The listing builds one solid part. Answer for the finished solid, in the listing's coordinates (mm). Face numbers are marked on the shaded views. A direction names the side the tool comes from. Round coordinates to 2 decimals unless told otherwise and drop trailing zeros. Loops run counter-clockwise (first coordinate to the right, second up) from the corner with the lowest first, then second, coordinate; pieces in that order, holes last. Notation, with made-up numbers: (48.5, -6.5) - (58.5, -6.5) arc R22 ccw to (58.5, 28.5) - close; hole circle Ø3 at (-33, 55). An arc over 180 degrees is marked (long way). One line per question, with ' | ' between items. Start each with the question number.
from build123d import *

# Parameters (mm, degrees)
ESBO_O1_W                = 15.15
ESBO_O1_H                = 30.65
ESBO_O1_R                = 1.55
RESSALTO_EXTRUS_O1_DEPTH = 1.55
ESBO_O2_W                = 6.85
ESBO_O2_H                = 6.85
RESSALTO_EXTRUS_O2_DEPTH = 6.45
ESBO_O3_R                = 1.65
CORTE_EXTRUS_O1_DEPTH    = 0.5
ESBO_O4_W                = 7.3
ESBO_O4_H                = 2.5
RESSALTO_EXTRUS_O3_DEPTH = 4.05
RESSALTO_EXTRUS_O5_DEPTH = 7.398508
ESBO_O12_W               = 1.34798559
ESBO_O12_H               = 5.991047065
ESBO_O12_W_2             = 0.998507844
ESBO_O12_W_3             = 2
CORTE_EXTRUS_O2_DEPTH    = 10
ESBO_O9_R                = 1.55
CORTE_EXTRUS_O3_DEPTH    = 0.1
RESSALTO_EXTRUS_O6_DEPTH = 1.9
ESBO_O18_R               = 0.297205441
ESBO_O18_R_2             = 0.285630525
RESSALTO_EXTRUS_O7_DEPTH = 0.2
ESBO_O25_R               = 0.285630525


with BuildPart() as part:
    # Esboço1 → Ressalto-extrusão1 (new body)
    with BuildSketch(Plane.XY):
        Rectangle(ESBO_O1_W, ESBO_O1_H)
        with Locations(Location((0, -6.025, 0), (0, 0, 180))):
            Circle(ESBO_O1_R, mode=Mode.SUBTRACT)
    extrude(amount=RESSALTO_EXTRUS_O1_DEPTH)

    # Esboço2 → Ressalto-extrusão2 (add)
    with BuildSketch(Plane.XY):
        with Locations((3.95, 1.7)):
            Rectangle(ESBO_O2_W, ESBO_O2_H)
    extrude(amount=RESSALTO_EXTRUS_O2_DEPTH)

    # Esboço3 → Corte-extrusão1 (cut)
    with BuildSketch(Plane.XY.offset(6.45)):
        with Locations((3.95, 1.7)):
            Circle(ESBO_O3_R)
        with BuildLine():
            Line((3.7, 1.95), (2.420294146, 1.95))
            ThreePointArc((2.420294146, 1.95), (2.853984489, 2.796015511), (3.7, 3.229705854))
            Line((3.7, 3.229705854), (3.7, 1.95))
        make_face(mode=Mode.SUBTRACT)
        with BuildLine():
            Line((5.479705854, 1.45), (4.2, 1.45))
            Line((4.2, 1.45), (4.2, 0.170294146))
            ThreePointArc((4.2, 0.170294146), (5.046015511, 0.603984489), (5.479705854, 1.45))
        make_face(mode=Mode.SUBTRACT)
        with BuildLine():
            Line((5.479705854, 1.95), (4.2, 1.95))
            Line((4.2, 1.95), (4.2, 3.229705854))
            ThreePointArc((4.2, 3.229705854), (5.046015511, 2.796015511), (5.479705854, 1.95))
        make_face(mode=Mode.SUBTRACT)
        with BuildLine():
            Line((3.7, 1.45), (3.7, 0.170294146))
            ThreePointArc((3.7, 0.170294146), (2.853984489, 0.603984489), (2.420294146, 1.45))
            Line((2.420294146, 1.45), (3.7, 1.45))
        make_face(mode=Mode.SUBTRACT)
    extrude(amount=-CORTE_EXTRUS_O1_DEPTH, mode=Mode.SUBTRACT)

    # Esboço4 → Ressalto-extrusão3 (add)
    with BuildSketch(Plane.XY):
        with Locations((0, -13.975)):
            Rectangle(ESBO_O4_W, ESBO_O4_H)
    extrude(amount=RESSALTO_EXTRUS_O3_DEPTH)

    # Esboço11 → Ressalto-extrusão5 (add)
    with BuildSketch(Plane.ZY.offset(3.65)):
        with BuildLine():
            Line((4.05, -14.175), (4.467357012, -14.175))
            ThreePointArc((4.467357012, -14.175), (4.679489046, -14.262867966), (4.767357012, -14.475))
            Line((4.767357012, -14.475), (4.767357012, -18.595051461))
            Line((4.767357012, -18.595051461), (5.167357012, -18.595051461))
            Line((5.167357012, -18.595051461), (5.167357012, -14.475))
            ThreePointArc((5.167357012, -14.475), (4.962331759, -13.980025253), (4.467357012, -13.775))
            Line((4.467357012, -13.775), (4.05, -13.775))
            Line((4.05, -13.775), (4.05, -14.175))
        make_face()
    extrude(amount=-RESSALTO_EXTRUS_O5_DEPTH)

    # Esboço12 → Corte-extrusão2 (cut)
    with BuildSketch(Plane.XY.offset(4.05)):
        with Locations((-3.423992795, -16.372351479)):
            Rectangle(ESBO_O12_W, ESBO_O12_H)
        with Locations((3.249253922, -16.372351479)):
            Rectangle(ESBO_O12_W_2, ESBO_O12_H)
        with Locations((-1.25, -16.372351479)):
            Rectangle(ESBO_O12_W_3, ESBO_O12_H)
        with Locations((1.25, -16.372351479)):
            Rectangle(ESBO_O12_W_3, ESBO_O12_H)
    extrude(amount=CORTE_EXTRUS_O2_DEPTH, mode=Mode.SUBTRACT)

    # Esboço9 → Corte-extrusão3 (cut)
    with BuildSketch(Plane.XY.offset(6.45)):
        with Locations((3.95, 1.7)):
            Circle(ESBO_O9_R)
    extrude(amount=-CORTE_EXTRUS_O3_DEPTH, mode=Mode.SUBTRACT)



with BuildPart() as body_2:
    # Esboço17 → Ressalto-extrusão6 (new body)
    with BuildSketch(Plane(origin=(0, 22.325, 0), x_dir=(1, 0, 0), z_dir=(0, 1, 0))):
        with BuildLine():
            Line((-1.446547614, -0.9), (1.446547614, -0.9))
            ThreePointArc((1.446547614, -0.9), (2.55, -3), (1.446547614, -5.1))
            Line((1.446547614, -5.1), (-1.446547614, -5.1))
            ThreePointArc((-1.446547614, -5.1), (-2.55, -3), (-1.446547614, -0.9))
        make_face()
    extrude(amount=RESSALTO_EXTRUS_O6_DEPTH)

    # Esboço18 → Ressalto-extrusão7 (add)
    with BuildSketch(Plane(origin=(0, 24.225, 0), x_dir=(1, 0, 0), z_dir=(0, 1, 0))):
        with Locations(Location((1.7, -3, 0), (0, 0, 180))):
            Circle(ESBO_O18_R)
        with Locations(Location((-1.7, -3, 0), (0, 0, 180))):
            Circle(ESBO_O18_R_2)
    extrude(amount=RESSALTO_EXTRUS_O7_DEPTH)


with BuildPart() as part_1:
    add(part.part)

    add(body_2.part)  # Varredura5 merges body 2
    # Varredura5: sweep along a path in Esboço19
    with BuildLine(Plane.ZY.offset(1.7)) as varredura5_path:
        Line((3, 22.325), (3, 15.227434518))
        ThreePointArc((3, 15.227434518), (2.707106781, 14.520327737), (2, 14.227434518))
        Line((2, 14.227434518), (1.55, 14.227434518))
    # Esboço25 → Varredura5 (sweep)
    with BuildSketch(Plane.XZ.offset(-22.325)):
        with Locations((-1.7, 3)):
            Circle(ESBO_O25_R)
    varredura5 = sweep(path=varredura5_path.line)

    # Espelhar1: Varredura5 across plane
    add(varredura5.mirror(Plane.ZY))


solid = part_1.part
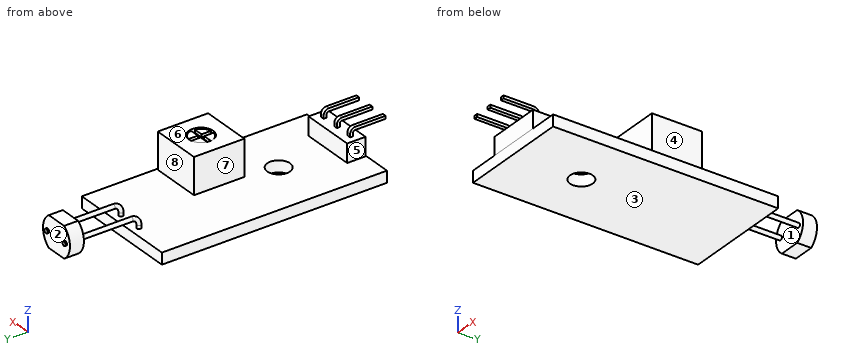
(1) Consider L1, parallel to Y at x = 1, z = 2 (3 decimals); L2, parallel to Y at x = 0, z = 1.25 (3 decimals); L3, parallel to Y at x = 0, z = 0.8 (3 decimals). Determine where each line is inside the solid, lowest interval first.
(2) A tool of negligible diameter and unlimited length cuts with its end or side. For the marked faces 4, 5, 6, 7 and 8, from which of +Z, -Z, +X, -X, +Y, -Y can it reach the whole face along a straight path? Write none if from no direction.
(3) Each of these flat-tipped pins is pushed along its axis until it touches: P1, Ø0.6, axis at y = -17, z = 4.5, coming from the -X side; P2, Ø2, axis at x = 0, z = 3, coming from the -Y side (3 decimals); P3, Ø5, axis at x = -0.5, y = 9, coming from the +Z side. Where does it stop, or does it pass through?
(4) Determine the mould class of the marked faces 1, 2 and 3 for opening direction Y: pulls with the +Y half, pulls with the -Y half, needs draft (parallel to the pull), parting line crosses it, or undercut.
(5) Find section B-B on y = -12. Write down the section's boundary in (x, z) (3 decimals).
(6) Find section A-A on y = -6.5. Write down the section's boundary in (x, z) (3 decimals).
Answer below:
1) L1: -15.225 to -12.725, -1.725 to 5.125, 22.325 to 24.225 | L2: -15.325 to -7.575, -4.475 to 15.325, 22.325 to 24.225 | L3: -15.325 to -7.575, -4.475 to 15.325
2) face 4: +Z, +X, +Y, -Y | face 5: +Z, -X, +Y, -Y | face 6: +Z, +X, -X, +Y, -Y | face 7: +Z, -X | face 8: +Z, +X, -X
3) P1: x = -2.75 | P2: y = -15.225 | P3: z = 1.55
4) face 1: undercut | face 2: pulls with the +Y half | face 3: needs draft
5) outline: (-7.575, 0) - (7.575, 0) - (7.575, 1.55) - (-7.575, 1.55) - close
6) outline: (-7.575, 0) - (-1.475, 0) - (-1.475, 1.55) - (-7.575, 1.55) - close; (1.475, 0) - (7.575, 0) - (7.575, 1.55) - (1.475, 1.55) - close
